Geometry: final body of the model. Coordinates: model frame, mm. Give positions to 0.01 mm unless a question says otherwise; leave off trailing zeros. Write each loop counter-clockwise with the first axis right and the second up, starting at its lowest first coordinate (ties: lowest second). Pieces come first, ordered by that corner, then holes. Notation, with made-up numbers: (83.25, 12.5) - (108.25, 12.5) arc R24 cw to (108.25, 22.5) - close; hole circle Ø2 at (-7, -5.75). An arc over 180 degrees is marked (long way). Return JSON: item names as keys, results as strings.
from build123d import *

# Parameters (mm, degrees)
SKETCH1_R           = 3.95
SKETCH1_R_2         = 1.475
SKETCH1_R_3         = 22.5
SKETCH1_R_4         = 2.4
SKETCH1_R_5         = 1.975
BOSS_EXTRUDE1_DEPTH = 5


with BuildPart() as part:
    # Sketch1 → Boss-Extrude1 (new body)
    with BuildSketch(Plane.XY):
        with BuildLine():
            Line((35, 0), (35, 162))
            ThreePointArc((35, 162), (0, 197), (-35, 162))
            Line((-35, 162), (-35, 0))
            ThreePointArc((-35, 0), (0, -35), (35, 0))
        make_face()
        Circle(SKETCH1_R, mode=Mode.SUBTRACT)
        with Locations((0, 29)):
            Circle(SKETCH1_R_2, mode=Mode.SUBTRACT)
        with Locations((0, 162)):
            Circle(SKETCH1_R_3, mode=Mode.SUBTRACT)
        with Locations((0, 133)):
            Circle(SKETCH1_R_2, mode=Mode.SUBTRACT)
        with Locations((-30, 97)):
            Circle(SKETCH1_R_2, mode=Mode.SUBTRACT)
        with Locations((30, 97)):
            Circle(SKETCH1_R_2, mode=Mode.SUBTRACT)
        with Locations((29, 0)):
            Circle(SKETCH1_R_2, mode=Mode.SUBTRACT)
        with Locations((0, -29)):
            Circle(SKETCH1_R_2, mode=Mode.SUBTRACT)
        with Locations((-29, 0)):
            Circle(SKETCH1_R_2, mode=Mode.SUBTRACT)
        with Locations((0, 12)):
            Circle(SKETCH1_R_4, mode=Mode.SUBTRACT)
        with Locations((12, 0)):
            Circle(SKETCH1_R_4, mode=Mode.SUBTRACT)
        with Locations((0, -12)):
            Circle(SKETCH1_R_4, mode=Mode.SUBTRACT)
        with Locations((-12, 0)):
            Circle(SKETCH1_R_4, mode=Mode.SUBTRACT)
        with Locations((0, 191)):
            Circle(SKETCH1_R_5, mode=Mode.SUBTRACT)
        with Locations((29, 162)):
            Circle(SKETCH1_R_5, mode=Mode.SUBTRACT)
        with Locations((-29, 162)):
            Circle(SKETCH1_R_5, mode=Mode.SUBTRACT)
        with Locations((-18.45, 110)):
            Circle(SKETCH1_R_2, mode=Mode.SUBTRACT)
        with Locations((-28.5, 35)):
            Circle(SKETCH1_R_2, mode=Mode.SUBTRACT)
        with Locations((-23.5, 35)):
            Circle(SKETCH1_R_2, mode=Mode.SUBTRACT)
        with Locations((-18.5, 35)):
            Circle(SKETCH1_R_2, mode=Mode.SUBTRACT)
        with Locations((-13.5, 35)):
            Circle(SKETCH1_R_2, mode=Mode.SUBTRACT)
        with Locations((-28.5, 40)):
            Circle(SKETCH1_R_2, mode=Mode.SUBTRACT)
        with Locations((-23.5, 40)):
            Circle(SKETCH1_R_2, mode=Mode.SUBTRACT)
        with Locations((-18.5, 40)):
            Circle(SKETCH1_R_2, mode=Mode.SUBTRACT)
        with Locations((-13.5, 40)):
            Circle(SKETCH1_R_2, mode=Mode.SUBTRACT)
        with Locations((-28.5, 45)):
            Circle(SKETCH1_R_2, mode=Mode.SUBTRACT)
        with Locations((-23.5, 45)):
            Circle(SKETCH1_R_2, mode=Mode.SUBTRACT)
        with Locations((-18.5, 45)):
            Circle(SKETCH1_R_2, mode=Mode.SUBTRACT)
        with Locations((-13.5, 45)):
            Circle(SKETCH1_R_2, mode=Mode.SUBTRACT)
        with Locations((-28.5, 50)):
            Circle(SKETCH1_R_2, mode=Mode.SUBTRACT)
        with Locations((-23.5, 50)):
            Circle(SKETCH1_R_2, mode=Mode.SUBTRACT)
        with Locations((-18.5, 50)):
            Circle(SKETCH1_R_2, mode=Mode.SUBTRACT)
        with Locations((-13.5, 50)):
            Circle(SKETCH1_R_2, mode=Mode.SUBTRACT)
        with BuildLine():
            Line((4.5, 80), (4.5, 40))
            ThreePointArc((4.5, 40), (0, 35.5), (-4.5, 40))
            Line((-4.5, 40), (-4.5, 80))
            ThreePointArc((-4.5, 80), (0, 84.5), (4.5, 80))
        make_face(mode=Mode.SUBTRACT)
        with BuildLine():
            Line((21.5, 80), (21.5, 40))
            ThreePointArc((21.5, 40), (17, 35.5), (12.5, 40))
            Line((12.5, 40), (12.5, 80))
            ThreePointArc((12.5, 80), (17, 84.5), (21.5, 80))
        make_face(mode=Mode.SUBTRACT)
        with BuildLine():
            Line((-16.95, 127.5), (-16.95, 122.5))
            ThreePointArc((-16.95, 122.5), (-18.45, 121), (-19.95, 122.5))
            Line((-19.95, 122.5), (-19.95, 127.5))
            ThreePointArc((-19.95, 127.5), (-18.45, 129), (-16.95, 127.5))
        make_face(mode=Mode.SUBTRACT)
    extrude(amount=BOSS_EXTRUDE1_DEPTH)


solid = part.part
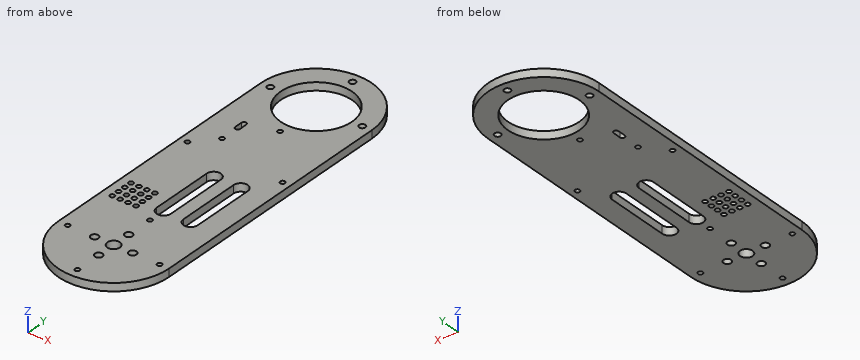
Q1. Section query A-A, the plane y = 72.5. Return the cut outline in (x, z), plus the area to 3 significant figures.
Answer key:
{"outline": "(-35, 0) - (-4.5, 0) - (-4.5, 5) - (-35, 5) - close; (4.5, 0) - (12.5, 0) - (12.5, 5) - (4.5, 5) - close; (21.5, 0) - (35, 0) - (35, 5) - (21.5, 5) - close", "area": "260 mm^2"}
Q2. Pin query (flat end, axial travel): P1, Ø2, axis at y = 170.5, z = 3, coming from the +X side; P2, Ø3, axis at x = 29, y = 162, coming from the -Z side; P3, Ø12.5, axis at x = 0, y = 0, coming from the +Z side; P4, Ø1.5, axis at x = -13, z = 3, coming from the -Y side. Return the tip coordinate at first contact, or that it passes through.
Answer key:
{"P1": "stops at x = 34.19", "P2": "passes through", "P3": "stops at z = 5", "P4": "stops at y = -32.79"}
Q3. Section query B-B, the plane x = 6.5. Return the cut outline in (y, z).
Answer key:
{"outline": "(-34.39, 0) - (140.46, 0) - (140.46, 5) - (-34.39, 5) - close; (183.54, 0) - (196.39, 0) - (196.39, 5) - (183.54, 5) - close"}
Q4. Section query C-C, the plane z = 0.85. Count the separate pieces of the cut face and the enclosed holes in it, plus the area to 3 significant figures.
Answer key:
{"separate pieces": "1", "enclosed holes": "36", "area": "12,400 mm^2"}
Q5. Material intervals for probe 1 along Y at (x, z) = (-24.5, 1.95) (3 decimals); probe 2 along Y at (x, z) = (-8, 0.75); probe 3 along Y at (x, z) = (-5, 2.4), sorted ascending. Write a range as [from, to].
Answer key:
{"probe 1": "y = [-24.995, 33.916], [36.084, 38.916], [41.084, 43.916], [46.084, 48.916], [51.084, 186.995]", "probe 2": "y = [-34.07, 140.97], [183.03, 196.07]", "probe 3": "y = [-34.64, 140.06], [183.94, 196.64]"}
